from build123d import *

# Parameters (mm, degrees)
F0_W = 3.1060343608
F0_H = 4.1245449741


with BuildPart() as f1:
    # F0 (on Top) → F1 (revolve)
    with BuildSketch(Plane.XY):
        Polygon((-75.8681371808, -68.3808345637), (-75.8681371808, -75.2311423421), (0, -75.2311423421), (0, -68.3808345637), (-65.233618021, -68.3808345637), align=None)
        Polygon((-65.233618021, -68.3808345637), (0, -68.3808345637), (0, -61.2551711489), (-56.3006289303, -61.2551711489), (-65.233618021, -61.2551711489), align=None)
        Polygon((-56.3006289303, -61.2551711489), (0, -61.2551711489), (0, -53.0980758273), (-46.5168766677, -53.0980758273), (-56.3006289303, -53.0980758273), align=None)
        Polygon((-46.5168766677, -53.0980758273), (0, -53.0980758273), (0, -46.3767246723), (-40.0174387131, -46.3767246723), (-46.5168766677, -46.3767246723), align=None)
        Polygon((-40.0174387131, -46.3767246723), (0, -46.3767246723), (0, -38.8292317048), (-25.3592459775, -38.8292317048), (-40.0174387131, -38.8292317048), align=None)
        Polygon((-25.3592459775, -38.8292317048), (0, -38.8292317048), (0, -31.9099235999), (-16.3148548454, -31.9099235999), (-25.3592459775, -31.9099235999), align=None)
        Polygon((-16.3148548454, -31.9099235999), (0, -31.9099235999), (0, -23.8791607417), (-8.1574274227, -23.8791607417), (-16.3148548454, -23.8791607417), align=None)
        Polygon((-8.1574274227, -23.8791607417), (0, -23.8791607417), (0, -15.3151774863), (-6.2120687217, -15.3151774863), (-8.1574274227, -15.3151774863), align=None)
        with Locations((-1.5530171804, -7.6774568423)):
            Rectangle(F0_W, F0_H)
        Polygon((-6.2120687217, -15.3151774863), (0, -15.3151774863), (0, -9.7397293293), (-3.1060343608, -9.7397293293), (-6.2120687217, -9.7397293293), align=None)
    revolve(axis=Axis((0, -71.8059884529, 0), (0, 1, 0)))


solid = f1.part
Design review of the part built by this model. Coordinates are the model's own, in mm. A direction names the side the tool comes from. Coordinates: 2 decimals unless noted, no trailing zeros. Order: outer loops, then holes, each group sorted by start corner. A loop starts at its lowest first (then second) coordinate and runs counter-clockwise, first axis right, second up.
Item 1: Take a section at A-A, the plane x = -37. Write out the cut boundary in (y, z).
Item 2: For line 1 (Y direction, x = -67.5, z = -26); line 2 (Y direction, x = -48.5, z = -5); line 3 (Z direction, x = 6, y = -16), list the stretches that pass through material, from the lowest coordinate up.
Item 3: Take a section at B-B, the plane y = -48.5. Write out the cut boundary in (x, z).
Item 4: Take a section at C-C, the plane z = 19.5. Write out the cut boundary in (x, y).
Item 5: Take a section at D-D, the plane z = -34. Write out the cut boundary in (x, y), then the cut area to 3 significant figures.
Item 6: For faces 1 (the flat face through (1, -75.231, 1)), 2 (the flat face through (2.4, -15.315, -6)), list the 3-axis set-ups (+Z, -Z, +X, -X, +Y, -Y) from which the entire face can be reached by the end or side of a thin tool; tool diameter is ignored.
Item 7: For pin 1 Ø3 at (y, z) = (-32, -19.5) entering from -X; pin 2 Ø3 at (x, z) = (-2, -17.5) entering from +Y; pin 3 Ø4 at (x, z) = (-52, 20.5) entering from +Y; pin 4 Ø13 at (x, z) = (2, 4) entering from +Y, all flat-tipped, find the tip position at first contact; note any pin that passes through.
The answers:
1. outline: (-75.23, -66.23) - (-68.38, -66.23) - (-68.38, -53.73) - (-61.26, -53.73) - (-61.26, -42.44) - (-53.1, -42.44) - (-53.1, -28.19) - (-46.38, -28.19) - (-46.38, -15.24) - (-38.83, -15.24) - (-38.83, 15.24) - (-46.38, 15.24) - (-46.38, 28.19) - (-53.1, 28.19) - (-53.1, 42.44) - (-61.26, 42.44) - (-61.26, 53.73) - (-68.38, 53.73) - (-68.38, 66.23) - (-75.23, 66.23) - close
2. line 1: y = -75.23 to -68.38
2. line 2: y = -75.23 to -53.1
2. line 3: z = -5.53 to 5.53
3. outline: circle Ø93.03 at (0, 0)
4. outline: (-73.32, -75.23) - (73.32, -75.23) - (73.32, -68.38) - (62.25, -68.38) - (62.25, -61.26) - (52.82, -61.26) - (52.82, -53.1) - (42.23, -53.1) - (42.23, -46.38) - (34.94, -46.38) - (34.94, -38.83) - (16.21, -38.83) - (16.21, -31.91) - (-16.21, -31.91) - (-16.21, -38.83) - (-34.94, -38.83) - (-34.94, -46.38) - (-42.23, -46.38) - (-42.23, -53.1) - (-52.82, -53.1) - (-52.82, -61.26) - (-62.25, -61.26) - (-62.25, -68.38) - (-73.32, -68.38) - close
5. outline: (-67.82, -75.23) - (67.82, -75.23) - (67.82, -68.38) - (55.67, -68.38) - (55.67, -61.26) - (44.87, -61.26) - (44.87, -53.1) - (31.75, -53.1) - (31.75, -46.38) - (21.1, -46.38) - (21.1, -38.83) - (-21.1, -38.83) - (-21.1, -46.38) - (-31.75, -46.38) - (-31.75, -53.1) - (-44.87, -53.1) - (-44.87, -61.26) - (-55.67, -61.26) - (-55.67, -68.38) - (-67.82, -68.38) - close
5. area: 3,200 mm2
6. face 1: +Z, -Z, +X, -X, -Y
6. face 2: +Y
7. pin 1: stops at x = -17.86
7. pin 2: stops at y = -23.88
7. pin 3: stops at y = -53.1
7. pin 4: stops at y = -5.62
